Can you work these out from the drawing? Everything is in mm from the part's minimum corner. Give positions to 0.01 mm unless a question says otherwise; leave off trailing zeros. Write each loop counter-clockwise with the first axis right and the second up, starting at its lowest first coordinate (ties: lowest second). Pieces come first, ordered by that corner, then holes. Notation, with made-up numbers: (64.5, 31.25) -> (74.5, 31.25) arc R26 ccw to (74.5, 54.25) -> close; hole circle Ø2 at (-7.5, 83.5). An arc over 180 degrees is marked (long way). Answer as CSV lines item,"result". Start each with the question number.
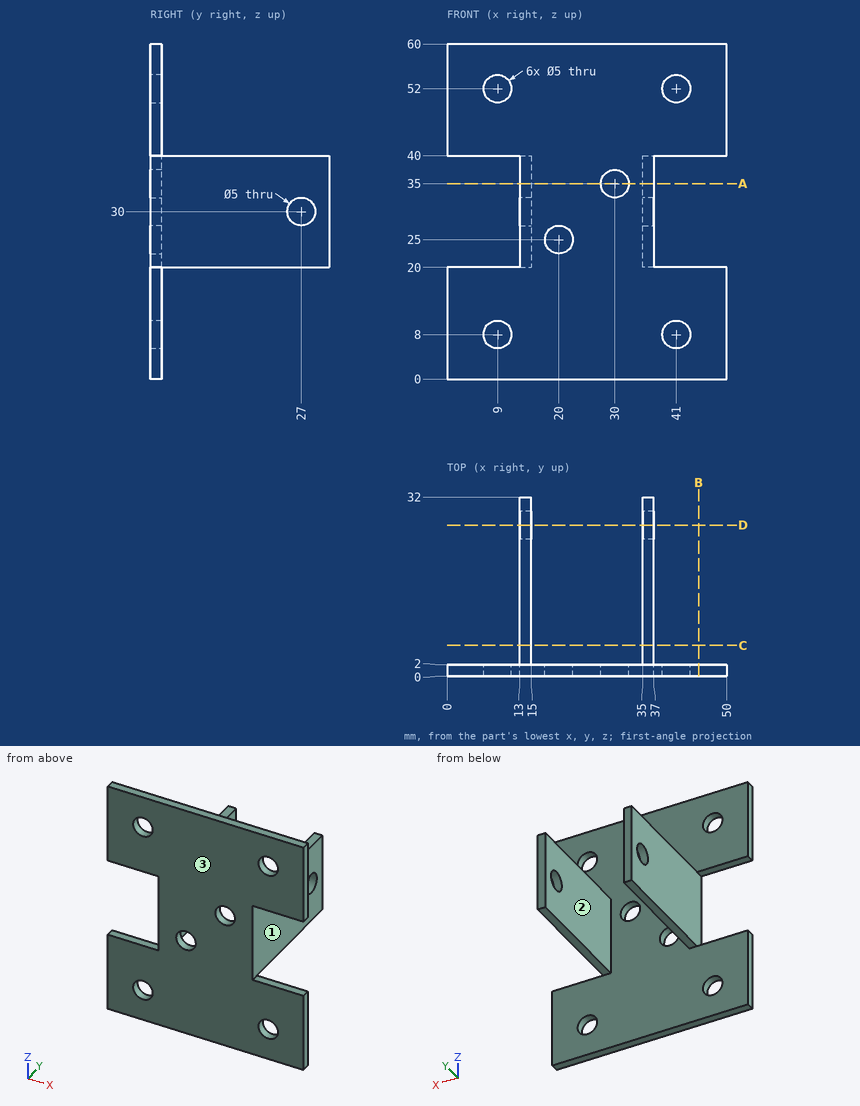
Item 1: If I drill on line 1 (X direction, y = 1, z = 52); line 2 (X direction, y = 8, z = 39); line 3 (Z direction, x = 36, y = 27), over which ranges is the centre line in solid material (lowest first)? Write a range as [from, to].
Item 2: If we section it at B-B (x = 45): Please give me the cut outline in (y, z).
Item 3: If we section it at D-D (y = 27): Please give me the cut outline in (x, z), and give its area (3 significant figures).
Item 4: If we section it at A-A (z = 35): Please give me the cut outline in (x, y), and give its area (3 significant figures).
Item 5: If we section it at C-C (y = 5.5): Please give me the cut outline in (x, z).
Item 6: I'm going to push flat-ended pins straight in: pin 1 (3 mm diameter, centred on x = 44, z = 50.5, fed in from +Y); pin 2 (0.6 mm diameter, centred on x = 35.5, y = 19.5, fed in from +Z); pin 3 (1.6 mm diameter, centred on x = 36, y = 24.5, fed in from -Z). Where does each tip first touch, or does it pass through?
Item 7: We'd pull the mould along X, two halves only. Please class the marked faces 1, 2 and 3: released by +X, released by -X, zero draft, split by the parting line, or undercut.
Final values:
1,line 1,"[0, 6.5], [11.5, 38.5], [43.5, 50]"
1,line 2,"[13, 15], [35, 37]"
1,line 3,"[20, 27.5], [32.5, 40]"
2,outline,"(0, 0) -> (2, 0) -> (2, 20) -> (0, 20) -> close; (0, 40) -> (2, 40) -> (2, 60) -> (0, 60) -> close"
3,outline,"(13, 20) -> (15, 20) -> (15, 27.5) -> (13, 27.5) -> close; (13, 32.5) -> (15, 32.5) -> (15, 40) -> (13, 40) -> close; (35, 20) -> (37, 20) -> (37, 27.5) -> (35, 27.5) -> close; (35, 32.5) -> (37, 32.5) -> (37, 40) -> (35, 40) -> close"
3,area,"60.0 mm2"
4,outline,"(13, 0) -> (27.5, 0) -> (27.5, 2) -> (15, 2) -> (15, 32) -> (13, 32) -> close; (32.5, 0) -> (37, 0) -> (37, 32) -> (35, 32) -> (35, 2) -> (32.5, 2) -> close"
4,area,"158 mm2"
5,outline,"(13, 20) -> (15, 20) -> (15, 40) -> (13, 40) -> close; (35, 20) -> (37, 20) -> (37, 40) -> (35, 40) -> close"
6,pin 1,"y = 2"
6,pin 2,"z = 40"
6,pin 3,"z = 20"
7,face 1,"released by +X"
7,face 2,"undercut"
7,face 3,"zero draft"
